Geometry check sheet. Reference: the model listing, model coordinates, mm. A direction names the side the tool comes from. Round coordinates to 2 decimals unless told otherwise and drop trailing zeros. Write each loop counter-clockwise with the first axis right and the second up, starting at its lowest first coordinate (ties: lowest second). Pieces come first, ordered by that corner, then holes.
Item 1: Cross-section at B-B (y = 6). Enter the section's corners in (x, z).
Item 2: Scan lines: probe 1 along Z at (x, y) = (7.75, 1.25); probe 2 along Z at (x, y) = (7, 8.5); probe 3 along X at (y, z) = (8, -58). Record each from-to range of solid material in increasing order.
Item 3: Cross-section at A-A (z = -48). Enter the section's corners in (x, y) (3 decimals), then the cut area to 3 significant figures.
Item 4: Depth check by flat-ended pin: P1, Ø3, axis at x = 9.8, z = -80.26, coming from the +Y side; P2, Ø1.9, axis at x = 9.5, z = -36.5, coming from the +Y side. Enter the tip coordinate at first touch or a pass-through.
Item 5: Draft check along X on faces 1 (the face through (0, 5, -44)), 2 (the face through (10, 5, -88.9)), 3 (the face through (10, 6, -13.97)). Enter one of: pulls with the +X half, pulls with the -X half, needs draft (parallel to the pull), parting line crosses it, or undercut.
Item 6: Access from +Z, -Z, +X, -X, +Y, -Y to the whole of each face (thin tool, end or side, straight path). Record for faces 4 (the face through (6.629, 6, -44)), 5 (the face through (10, 5, 0)).
Item 7: Cross-section at C-C (x = 11.5). Enter the section's corners in (y, z) (3 decimals), then the cut area to 3 significant figures.
from build123d import *

# Parameters (mm, degrees)
SKETCH1_W                  = 19.6088
SKETCH1_H                  = 88.9
SKETCH1_R                  = 2.54
BOSS_EXTRUDE1_DEPTH        = 9.525
SKETCH2_W                  = 6.35
SKETCH2_H                  = 60.96
CUT_EXTRUDE1_DEPTH         = 6.477
F_10_32_TAPPED_HOLE4_D     = 5.1054
F_10_32_TAPPED_HOLE4_DEPTH = 16.51
F_10_32_TAPPED_HOLE4_TIP   = 1.533816902


with BuildPart() as part:
    # Sketch1 → Boss-Extrude1 (new body)
    with BuildSketch(Plane(origin=(0, 0, 0), x_dir=(1, 0, 0), z_dir=(0, 1, 0))):
        with Locations((9.8044, 44.45)):
            Rectangle(SKETCH1_W, SKETCH1_H)
        with Locations((9.8044, 80.264)):
            Circle(SKETCH1_R, mode=Mode.SUBTRACT)
        with Locations((9.8044, 8.636)):
            Circle(SKETCH1_R, mode=Mode.SUBTRACT)
    extrude(amount=BOSS_EXTRUDE1_DEPTH)

    # Sketch2 → Cut-Extrude1 (cut)
    with BuildSketch(Plane(origin=(0, 9.525, 0), x_dir=(1, 0, 0), z_dir=(0, 1, 0))):
        with Locations((9.8044, 44.45)):
            Rectangle(SKETCH2_W, SKETCH2_H)
    extrude(amount=-CUT_EXTRUDE1_DEPTH, mode=Mode.SUBTRACT)

    # #10-32 Tapped Hole4
    with Locations(Plane(origin=(0, 9.525, 0), x_dir=(1, 0, 0), z_dir=(0, 1, 0))):
        with Locations((9.8044, 80.264), (9.8044, 8.636)):
            Hole(F_10_32_TAPPED_HOLE4_D / 2, depth=F_10_32_TAPPED_HOLE4_DEPTH)
            with Locations((0, 0, -(F_10_32_TAPPED_HOLE4_DEPTH + F_10_32_TAPPED_HOLE4_TIP / 2))):  # 118° drill point
                Cone(0, F_10_32_TAPPED_HOLE4_D / 2, F_10_32_TAPPED_HOLE4_TIP, mode=Mode.SUBTRACT)


solid = part.part
Resolved:
1. outline: (0, -88.9) - (19.61, -88.9) - (19.61, 0) - (0, 0) - close; hole (6.63, -74.93) - (12.98, -74.93) - (12.98, -13.97) - (6.63, -13.97) - close; hole circle Ø5.11 at (9.8, -80.26); hole circle Ø5.11 at (9.8, -8.64)
2. probe 1: z = -88.9 to -81.78, -78.75 to -10.15, -7.12 to 0
2. probe 2: z = -88.9 to -74.93, -13.97 to 0
2. probe 3: x = 0 to 6.63, 12.98 to 19.61
3. outline: (0, 0) - (19.609, 0) - (19.609, 9.525) - (12.979, 9.525) - (12.979, 3.048) - (6.629, 3.048) - (6.629, 9.525) - (0, 9.525) - close
3. area: 146 mm2
4. P1: passes through
4. P2: stops at y = 3.05
5. face 1: pulls with the -X half
5. face 2: needs draft
5. face 3: undercut
6. face 4: +Y
6. face 5: +Z, +X, -X, +Y, -Y
7. outline: (0, -88.9) - (9.525, -88.9) - (9.525, -82.172) - (0, -82.172) - close; (0, -78.356) - (9.525, -78.356) - (9.525, -74.93) - (3.048, -74.93) - (3.048, -13.97) - (9.525, -13.97) - (9.525, -10.544) - (0, -10.544) - close; (0, -6.728) - (9.525, -6.728) - (9.525, 0) - (0, 0) - close
7. area: 379 mm2
